from build123d import *

# Parameters (mm, degrees)
SKETCH1_R             = 1.5
BOSS_EXTRUDE1_DEPTH   = 1.5
SKETCH2_R             = 2.25
BOSS_EXTRUDE2_DEPTH   = 1.5
BOSS_EXTRUDE2_2_DEPTH = 1.5
FILLET12_R            = 0.25
FILLET13_R            = 0.25
FILLET14_R            = 0.25


with BuildPart() as part:
    # Sketch1 → Boss-Extrude1 (new body)
    with BuildSketch(Plane.XY):
        with BuildLine():
            Line((-17.5, 10), (-17.386859967, 1.5))
            Line((-17.386859967, 1.5), (-9.886859967, 1.5))
            ThreePointArc((-9.886859967, 1.5), (-7.582875444, -6.519202405), (0, -10))
            Line((0, -10), (17.5, -10))
            Line((17.5, -10), (17.386859967, -1.5))
            Line((17.386859967, -1.5), (9.886859967, -1.5))
            ThreePointArc((9.886859967, -1.5), (7.582875444, 6.519202405), (0, 10))
            Line((0, 10), (-17.5, 10))
        make_face()
        Circle(SKETCH1_R, mode=Mode.SUBTRACT)
    extrude(amount=-BOSS_EXTRUDE1_DEPTH)

    # Fillet13
    fillet13_edges = [part.edges().sort_by_distance(p)[0] for p in [
        (13.636859967, -1.5, 0),
        (-8.75, 10, -1.5),
        (8.75, -10, 0),
        (-7.582875444, -6.519202405, 0),
        (-13.636859967, 1.5, 0),
        (-8.75, 10, 0),
        (7.582875444, 6.519202405, 0),
        (-13.636859967, 1.5, -1.5),
        (-7.582875444, -6.519202405, -1.5),
        (8.75, -10, -1.5),
        (13.636859967, -1.5, -1.5),
        (7.582875444, 6.519202405, -1.5),
    ]]
    fillet(fillet13_edges, radius=FILLET13_R)



with BuildPart() as body_2:
    # Sketch2 → Boss-Extrude2 (new body)
    with BuildSketch(Plane.XY):
        with BuildLine():
            Line((22.5, -1.520409702), (80.5, -1.520409702))
            ThreePointArc((80.5, -1.520409702), (84.75, -5.770409702), (80.5, -10.020409702))
            Line((80.5, -10.020409702), (22.5, -10.020409702))
            Line((22.5, -10.020409702), (22.5, -1.520409702))
        make_face()
        with Locations((80.5, -5.770409702)):
            Circle(SKETCH2_R, mode=Mode.SUBTRACT)
    extrude(amount=BOSS_EXTRUDE2_DEPTH)

    # Fillet12
    fillet12_edges = [body_2.edges().sort_by_distance(p)[0] for p in [
        (84.75, -5.770409702, 1.5),
        (51.5, -1.520409702, 1.5),
        (51.5, -1.520409702, 0),
        (84.75, -5.770409702, 0),
        (51.5, -10.020409702, 0),
        (51.5, -10.020409702, 1.5),
    ]]
    fillet(fillet12_edges, radius=FILLET12_R)


with BuildPart() as body_3:
    # Sketch2 → Boss-Extrude2 2 (new body)
    with BuildSketch(Plane.XY):
        with BuildLine():
            Line((-22.5, 10.120226545), (-80.5, 10.120226545))
            ThreePointArc((-80.5, 10.120226545), (-84.75, 5.870226545), (-80.5, 1.620226545))
            Line((-80.5, 1.620226545), (-22.5, 1.620226545))
            Line((-22.5, 1.620226545), (-22.5, 10.120226545))
        make_face()
        with Locations((-80.5, 5.870226545)):
            Circle(SKETCH2_R, mode=Mode.SUBTRACT)
    extrude(amount=BOSS_EXTRUDE2_2_DEPTH)

    # Fillet14
    fillet14_edges = [body_3.edges().sort_by_distance(p)[0] for p in [
        (-51.5, 10.120226545, 0),
        (-84.75, 5.870226545, 0),
        (-51.5, 1.620226545, 0),
        (-51.5, 10.120226545, 1.5),
        (-84.75, 5.870226545, 1.5),
        (-51.5, 1.620226545, 1.5),
    ]]
    fillet(fillet14_edges, radius=FILLET14_R)


with BuildPart() as part_1:
    add(part.part)

    add(body_2.part)  # loft3 joins it to this body
    # loft from a face of the part (loft3)
    loft([part_1.faces().sort_by_distance((17.443429983, -5.75, -0.75))[0], part_1.faces().sort_by_distance((22.5, -5.770409702, 0.75))[0]])


    add(body_3.part)  # loft4 joins it to this body
    # loft from a face of the part (loft4)
    loft([part_1.faces().sort_by_distance((-17.443429983, 5.75, -0.75))[0], part_1.faces().sort_by_distance((-22.5, 5.870226545, 0.75))[0]])


solid = part_1.part
Work out the finished part from the listing and answer in its coordinate system (mm). A direction names the side the tool comes from. Coordinates: 2 decimals unless noted, no trailing zeros. Write each loop counter-clockwise with the first axis right and the second up, starting at its lowest first coordinate (ties: lowest second). Pieces come first, ordered by that corner, then holes. Notation, with made-up numbers: M 41,89.25 L 96,89.25 A8 cw 96,96.25 Z; hole C 35,47 d7. An arc over 180 degrees is marked long. Answer as CSV lines item,"result". Start each with the question number.
Item 1: A tool of negligible diameter and unlimited length cuts with its end or side. For faces 1 (the face through (-54, 6, 1.5)), 2 (the face through (-54, 6, 0)), 3 (the face through (0, 2, -1.5)), 4 (the face through (0, 2, 0)), 5 (the face through (54, -6, 0)), from which of +Z, -Z, +X, -X, +Y, -Y can it reach the whole face along a straight path? Write none if from no direction.
Item 2: Flat-ended cylindrical pins translate along their axes: P1, Ø10, axis at x = -36, y = -8, coming from the -Z side; P2, Ø6.5, axis at x = 39, y = -7, coming from the -Z side; P3, Ø10, axis at x = -4, y = 1, coming from the +Z side; P4, Ø0.8, axis at x = 8, z = -0.5, coming from the -Y side. Find the tip coordinate at first contact, or state that the pin passes through.
Item 3: Consider L1, parallel to Y at x = 80.5, z = 1.1; L2, parallel to Z at x = -54, y = 5.25; L3, parallel to Y at x = 11, z = -0.5. Determine where each line is inside the solid, lowest interval first.
Item 4: Determine the mould class of faces 6 (the face through (-1.5, 0.07, -0.74)), 7 (the face through (-84.75, 5.96, 0.74)), 8 (the face through (84.75, -5.68, 0.74)), 9 (the face through (-78.354, 6.546, 0.74)) for opening direction X: released by +X, released by -X, zero draft, split by the parting line, or undercut.
Item 5: Section A-A on x = 24 is taken. Write down the section's boundary in (y, z), and give its area (3 significant figures).
Checks:
1,face 1,"+Z, +X, -X, +Y, -Y"
1,face 2,"-Z, -X, +Y, -Y"
1,face 3,"-Z, +X, -X, +Y, -Y"
1,face 4,"+Z, +Y, -Y"
1,face 5,"-Z, +X, +Y, -Y"
2,P1,"passes through"
2,P2,"stops at z = 0"
2,P3,"stops at z = 0"
2,P4,"stops at y = -10"
3,L1,"y = -10.02 to -8.02, -3.52 to -1.52"
3,L2,"z = 0 to 1.5"
3,L3,"y = -10 to -1.5"
4,face 6,"undercut"
4,face 7,"released by -X"
4,face 8,"released by +X"
4,face 9,"undercut"
5,outline,"M -10.02,0.25 A0.25 ccw -9.77,0 L -1.77,0 A0.25 ccw -1.52,0.25 L -1.52,1.25 A0.25 ccw -1.77,1.5 L -9.77,1.5 A0.25 ccw -10.02,1.25 Z"
5,area,"12.7 mm²"
